from build123d import *

# Parameters (mm, degrees)
F3_DEPTH = 2
F4_R     = 0.2
F5_SIZE  = 0.3


with BuildPart() as f1:
    # F0 (on Front) → F1 (revolve)
    with BuildSketch(Plane.XZ):
        Polygon((-2.75, 0), (0, 0), (0, 8), (-1.5, 8), (-1.5, 3), (-2.75, 3), align=None)
    revolve(axis=Axis((0, 0, 4), (0, 0, 1)))

    # F2 (on face) → F3 (cut)
    with BuildSketch(Plane(origin=(0, 0, 0), x_dir=(1, 0, 0), z_dir=(0, 0, -1))):
        Polygon((0.721688, 1.25), (-0.721688, 1.25), (-1.443376, 0), (-0.721688, -1.25), (0.721688, -1.25), (1.443376, 0), align=None)
    extrude(amount=-F3_DEPTH, mode=Mode.SUBTRACT)

    # F4
    f4_edges = [f1.edges().sort_by_distance(p)[0] for p in [
        (2.75, 0, 0),
        (2.75, 0, 3),
    ]]
    fillet(f4_edges, radius=F4_R)

    # F5
    f5_edges = [f1.edges().sort_by_distance(p)[0] for p in [
        (1.5, 0, 8),
    ]]
    chamfer(f5_edges, length=F5_SIZE)


solid = f1.part
For this review, take the finished solid that the model builds, in its own axes (mm). A direction names the side the tool comes from. Give positions to 0.01 mm unless a question says otherwise; leave off trailing zeros. Loops run counter-clockwise (first coordinate to the right, second up) from the corner with the lowest first, then second, coordinate; pieces in that order, holes last. Notation, with made-up numbers: M -23.75,-34.75 L 5.25,-34.75 A29 ccw 5.25,-4.75 Z; hole C 71,-34.5 d7. An arc over 180 degrees is marked long. Answer as a JSON object with one key per item and string values. Group by question number.
Q1. Add section B-B on z = 4.75. Give the boundary of the cut face in (x, y).
Q2. Mouldability with a two-part tool opening along Y and no side actions: class faces 4 (the flat face through (0, 1.25, 1)), 5 (the cylindrical face through (0.596, 2.685, 1.482)), 6 (the flat face through (0, 0, 8)) as +Y half, -Y half, draft (parallel to the pull), parting line (faces both ways), or undercut.
Q3. Tool access review of faces 1 (the cylindrical face through (1.5, -0.07, 5.32)), 2 (the flat face through (-1.1, 1.1, 0)), 3 (the flat face through (0, -1.25, 1)): name each direction out of +Z, -Z, +X, -X, +Y, -Y from which nothing blocks a thin tool from reaching the whole face with its end or side.
Q4. Insertion check: P1, Ø0.7, axis at x = 0.5, z = 1, coming from the -Y side; P2, Ø1.5, axis at y = -2, z = 2, coming from the +X side; P3, Ø0.8, axis at x = 0.5, y = 0, coming from the -Z side. Each pin has a flat end and moves straight along its axis. Give the tip position at first contact, or say it passes through.
Q5. Add section A-A on x = 0. Give the boundary of the cut face in (y, z), and give its area (3 significant figures).
Q6. For probe 1 along Y at (x, z) = (0.1, 7.75); probe 2 along Z at (x, y) = (2, 0.4); probe 3 along Y at (x, z) = (0.15, 1), list the stretches that pass through material, from the lowest coordinate up. Write a range as [from, to].
Checked values:
{
 "1": {"outline": "C 0,0 d3"},
 "2": {"face 4": "undercut", "face 5": "parting line", "face 6": "draft"},
 "3": {"face 1": "+Z", "face 2": "-Z, +X, -X, +Y, -Y", "face 3": "-Z"},
 "4": {"P1": "y = -2.75", "P2": "x = 2.45", "P3": "z = 2"},
 "5": {"outline": "M -2.75,0.2 A0.2 ccw -2.55,0 L -1.25,0 L -1.25,2 L 1.25,2 L 1.25,0 L 2.55,0 A0.2 ccw 2.75,0.2 L 2.75,2.8 A0.2 ccw 2.55,3 L 1.5,3 L 1.5,7.7 L 1.2,8 L -1.2,8 L -1.5,7.7 L -1.5,3 L -2.55,3 A0.2 ccw -2.75,2.8 Z", "area": "26.4 mm²"},
 "6": {"probe 1": "[-1.45, 1.45]", "probe 2": "[0, 3]", "probe 3": "[-2.75, -1.25], [1.25, 2.75]"}
}
